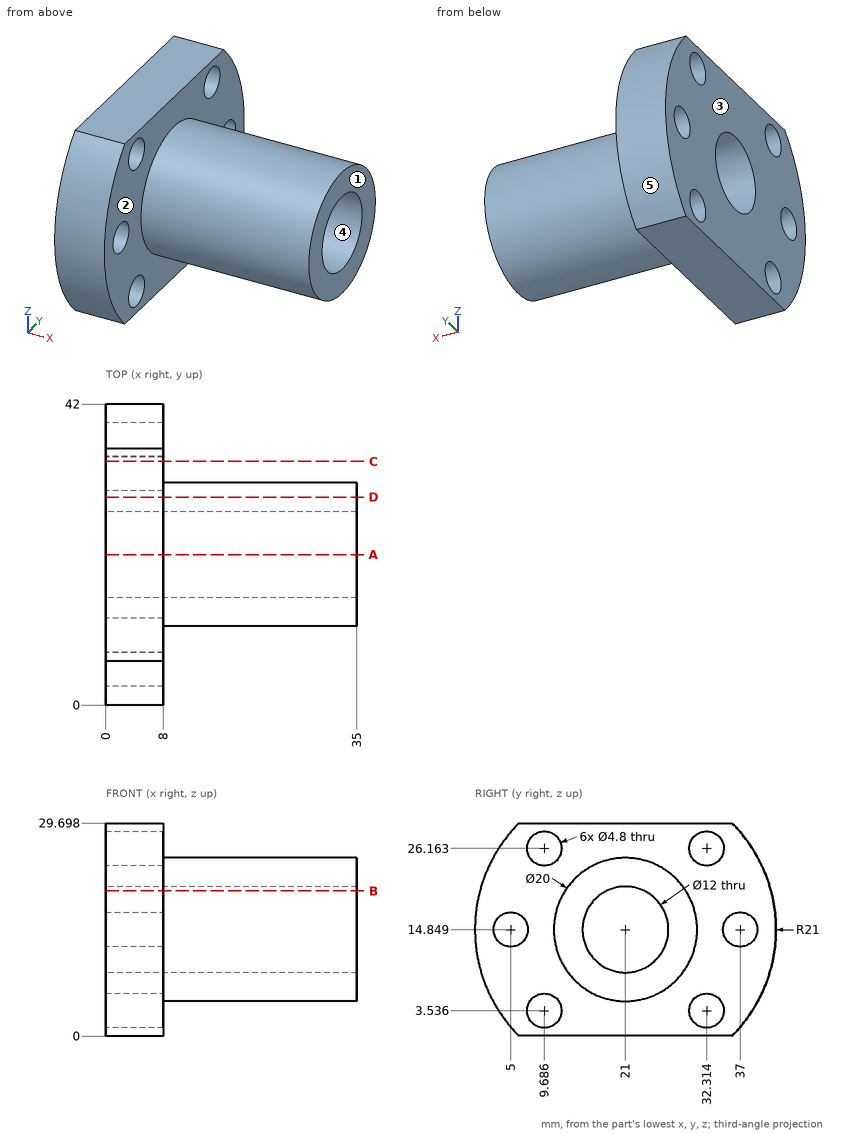
The figure shows three views and two pictorial views of one solid part (mm, origin at its lowest corner). Answer the questions. A direction names the side the tool comes from. Round coordinates to 2 decimals unless told otherwise and drop trailing zeros. Loops run counter-clockwise (first coordinate to the right, second up) from the corner with the lowest first, then second, coordinate; pieces in that order, holes last. Notation, with made-up numbers: M 18.5,-26.75 L 59.5,-26.75 A23 ccw 59.5,0.25 Z; hole C -15.5,-24 d11. An arc over 180 degrees is marked long. Write each question's results on one line, items separated by ' | '. Start each with the question number.
1) Find section D-D on y = 29. Write down the section's boundary in (x, z).
2) Each of these flat-tipped pins is pushed along its axis until it touches: pin 1 (6 mm diameter, centred on x = 25, z = 22.5, fed in from -Y); pin 2 (5.5 mm diameter, centred on y = 5, z = 14.85, fed in from +X); pin 3 (3 mm diameter, centred on x = 20, z = 3, fed in from -Y); pin 4 (1 mm diameter, centred on x = 19, y = 16, fed in from +Z). Where does it stop, or does it pass through?
3) Straight lines are drawn through the part: probe 1 along Y at (x, z) = (33.5, 14.5) (1 decimal); probe 2 along Z at (x, y) = (33.5, 21); probe 3 along Y at (x, z) = (6.5, 13.25) (1 decimal). For each, find the intervals that lie inside material, in ascending order.
4) Find section A-A on y = 21. Write down the section's boundary in (x, z).
5) Determine the mould class of the marked faces 3, 4 and 5 for opening direction Z: pulls with the +Z half, pulls with the -Z half, needs draft (parallel to the pull), parting line crosses it, or undercut.
6) Find section C-C on y = 34. Write down the section's boundary in (x, z) (1 decimal).
7) Which of the six approach directions +Z, -Z, +X, -X, +Y, -Y give full straight-line access (tool end or side, diameter ignored) to the marked faces 1 and 2?
8) Find section B-B on z = 20.25. Write down the section's boundary in (x, y).
Final values:
1) outline: M 0,0 L 8,0 L 8,8.85 L 35,8.85 L 35,20.85 L 8,20.85 L 8,29.7 L 0,29.7 Z
2) pin 1: y = 12.15 | pin 2: x = 8 | pin 3: through | pin 4: z = 23.78
3) probe 1: 11 to 15, 27 to 31 | probe 2: 4.85 to 8.85, 20.85 to 24.85 | probe 3: 0.1 to 3.2, 6.8 to 15.2, 26.8 to 35.2, 38.8 to 41.9
4) outline: M 0,0 L 8,0 L 8,4.85 L 35,4.85 L 35,8.85 L 0,8.85 Z; M 0,20.85 L 35,20.85 L 35,24.85 L 8,24.85 L 8,29.7 L 0,29.7 Z
5) face 3: needs draft | face 4: undercut | face 5: parting line crosses it
6) outline: M 0,0 L 8,0 L 8,1.8 L 0,1.8 Z; M 0,5.2 L 8,5.2 L 8,24.5 L 0,24.5 Z; M 0,27.9 L 8,27.9 L 8,29.7 L 0,29.7 Z
7) face 1: +Z, -Z, +X, +Y, -Y | face 2: +X
8) outline: M 0,0.71 L 8,0.71 L 8,12.58 L 35,12.58 L 35,18.39 L 0,18.39 Z; M 0,23.61 L 35,23.61 L 35,29.42 L 8,29.42 L 8,41.29 L 0,41.29 Z
